from build123d import *

# Parameters (mm, degrees)
F0_R     = 20
F0_R_2   = 10
F1_DEPTH = 20
F3_DEPTH = 25
F5_DEPTH = 20


with BuildPart() as f1:
    # F0 (on Front) → F1 (new body)
    with BuildSketch(Plane.XZ):
        Circle(F0_R)
        Circle(F0_R_2, mode=Mode.SUBTRACT)
    extrude(amount=F1_DEPTH)

    # F2 (on Right) → F3 (join, symmetric)
    with BuildSketch(Plane.YZ):
        Polygon((0, 16.390087), (0, 55.571124), (-18.135777, 16.390087), align=None)
    extrude(amount=F3_DEPTH, both=True)

    # F4 (on Right) → F5 (join, symmetric)
    with BuildSketch(Plane.YZ):
        Polygon((-17.94181, -19.881465), (0, -48.588365), (0, -19.881465), align=None)
    extrude(amount=F5_DEPTH, both=True)


solid = f1.part
The listing builds one solid part. Answer for the finished solid, in the listing's coordinates (mm). A direction names the side the tool comes from. Coordinates: 2 decimals unless noted, no trailing zeros. Write each loop counter-clockwise with the first axis right and the second up, starting at its lowest first coordinate (ties: lowest second). Pieces come first, ordered by that corner, then holes. Notation, with made-up numbers: (9.5, 60.5) - (24.5, 60.5) arc R26 cw to (24.5, 91.5) - close; hole circle Ø11 at (60, 22.25). An arc over 180 degrees is marked (long way). Return JSON: item names as keys, results as strings.
1. The part is cut by section A-A on z = 0. Determine the outline of the cut face in (x, y), then the cut area to 3 significant figures.
Final values:
{"outline": "(-20, -20) - (-10, -20) - (-10, 0) - (-20, 0) - close; (10, -20) - (20, -20) - (20, 0) - (10, 0) - close", "area": "400 mm^2"}
2. Which of the six approach directions +Z, -Z, +X, -X, +Y, -Y give full straight-line access (tool end or side, diameter ignored) to faces 1 (the face through (18, -9, 16.39)), 2 (the face through (-2.17, -9.86, -9.76)), 3 (the face through (20, -5, -28)), 4 (the face through (0.28, -9.1, -34.03)), 5 (the face through (-20, -5, -28))?
Final values:
{"face 1": "+X, +Y, -Y", "face 2": "+Y, -Y", "face 3": "-Z, +X, +Y, -Y", "face 4": "-Z, +X, -X, -Y", "face 5": "-Z, -X, +Y, -Y"}
3. The part is cut by section B-B on y = -12. Determine the outline of the cut face in (x, z).
Final values:
{"outline": "(-25, 16.39) - (-11.46, 16.39) arc R20 ccw to (-2.17, -19.88) - (-20, -19.88) - (-20, -29.39) - (20, -29.39) - (20, -19.88) - (2.17, -19.88) arc R20 ccw to (11.46, 16.39) - (25, 16.39) - (25, 29.65) - (-25, 29.65) - close; hole circle Ø20 at (0, 0)"}
4. The part is cut by section D-D on x = 0. Determine the outline of the cut face in (y, z).
Final values:
{"outline": "(-20, -20) - (-17.87, -20) - (0, -48.59) - (0, -10) - (-20, -10) - close; (-20, 10) - (0, 10) - (0, 55.57) - (-16.46, 20) - (-20, 20) - close"}
5. The part is cut by section C-C on x = -5. Determine the outline of the cut face in (y, z), then the cut area to 3 significant figures.
Final values:
{"outline": "(-20, -19.36) - (0, -19.36) - (0, -8.66) - (-20, -8.66) - close; (-20, 8.66) - (0, 8.66) - (0, 55.57) - (-16.76, 19.36) - (-20, 19.36) - close; (-17.94, -19.88) - (0, -48.59) - (0, -19.88) - close", "area": "989 mm^2"}
6. For a pull along Z with two mould halves and no side action, classify faces 6 (the face through (0.35, -8.941, 36.255)), 7 (the face through (11, -9, -19.881)), 8 (the face through (-5, -20, 9)) as +Z half, -Z half, draft (parallel to the pull), parting line (faces both ways), or undercut.
Final values:
{"face 6": "+Z half", "face 7": "undercut", "face 8": "draft"}
7. Consider line 1 along Z through (x, y) = (-18, -12.5); line 2 along Z through (x, y) = (-6, -9); line 3 along Z through (x, y) = (0, -8.75). Determine where each line is inside the solid, lowest interval first.
Final values:
{"line 1": "-28.59 to -19.88, -8.72 to 8.72, 16.39 to 28.57", "line 2": "-34.19 to -19.88, -19.08 to -8, 8 to 36.13", "line 3": "-34.59 to -10, 10 to 36.67"}
8. Each of these flat-tipped pins is pushed along its axis until it touches: pin 1 Ø5 at (x, y) = (-5, -14.5) entering from -Z; pin 2 Ø23 at (x, z) = (0, 0) entering from -Y; pin 3 Ø11 at (x, y) = (21.5, -10.5) entering from -Z; pin 4 Ø6 at (x, y) = (-15, -10) entering from +Z. Where does it stop, or does it pass through?
Final values:
{"pin 1": "z = -29.39", "pin 2": "y = -20", "pin 3": "z = -40.25", "pin 4": "z = 40.45"}
